Check sheet for the modelled part. Datum: model origin and axes. Units: mm. A direction names the side the tool comes from. Round coordinates to 2 decimals unless told otherwise and drop trailing zeros. Loops run counter-clockwise (first coordinate to the right, second up) from the corner with the lowest first, then second, coordinate; pieces in that order, holes last. Notation, with made-up numbers: (-2, 32.25) -> (24, 32.25) arc R5 cw to (24, 41.25) -> close; hole circle Ø7 at (64, 89.25). An arc over 180 degrees is marked (long way). Return JSON: item names as keys, results as strings.
from build123d import *

# Parameters (mm, degrees)
ESQUISSE1_W             = 49.5
ESQUISSE1_H             = 49.5
ESQUISSE1_W_2           = 43.5
ESQUISSE1_H_2           = 43.5
BOSS_EXTRU_1_DEPTH      = 30
ESQUISSE2_W             = 10
ESQUISSE2_H             = 10
ESQUISSE2_R             = 1.75
BOSS_EXTRU_2_DEPTH      = 5
CONG_1_R                = 1
CONG_2_R                = 3
CONG_3_R                = 1
CUT_EXTRUDE1_DEPTH      = 24
CUT_EXTRUDE1_DEPTH_BACK = 21.171554026
SKETCH1_W               = 3.5
SKETCH1_H               = 15


with BuildPart() as part:
    # Esquisse1 → Boss.-Extru.1 (new body)
    with BuildSketch(Plane.XY):
        with Locations((24.75, 24.75)):
            Rectangle(ESQUISSE1_W, ESQUISSE1_H)
        with Locations((24.75, 24.75)):
            Rectangle(ESQUISSE1_W_2, ESQUISSE1_H_2, mode=Mode.SUBTRACT)
    extrude(amount=BOSS_EXTRU_1_DEPTH)

    # Esquisse2 → Boss.-Extru.2 (add)
    # profile 1 of 2: a face of its own
    with BuildSketch(Plane(origin=(0, 0, 0), x_dir=(-1, 0, 0), z_dir=(0, 0, -1))):
        with Locations((-5, 54.5)):
            Rectangle(ESQUISSE2_W, ESQUISSE2_H)
        with Locations((-5, 54.5)):
            Circle(ESQUISSE2_R, mode=Mode.SUBTRACT)
    # profile 2 of 2: a face of its own
    with BuildSketch(Plane(origin=(0, 0, 0), x_dir=(-1, 0, 0), z_dir=(0, 0, -1))):
        with Locations((-44.5, -5)):
            Rectangle(ESQUISSE2_W, ESQUISSE2_H)
        with Locations((-44.5, -5)):
            Circle(ESQUISSE2_R, mode=Mode.SUBTRACT)
    extrude(amount=-BOSS_EXTRU_2_DEPTH)

    # Congé1
    cong_1_edges = [part.edges().sort_by_distance(p)[0] for p in [
        (0, 59.5, 2.5),
        (10, 59.5, 2.5),
        (49.5, -10, 2.5),
        (39.5, -10, 2.5),
        (49.5, 49.5, 15),
        (0, 0, 15),
    ]]
    fillet(cong_1_edges, radius=CONG_1_R)

    # Congé2
    cong_2_edges = [part.edges().sort_by_distance(p)[0] for p in [
        (10, 49.5, 2.5),
        (39.5, 0, 2.5),
    ]]
    fillet(cong_2_edges, radius=CONG_2_R)

    # Congé3
    cong_3_edges = [part.edges().sort_by_distance(p)[0] for p in [
        (6.5, 49.5, 5),
        (43, 0, 5),
    ]]
    fillet(cong_3_edges, radius=CONG_3_R)

    # Sketch1 → Cut-Extrude1 (cut, two sides: drawn at the far end of the back side and taken through both)
    with BuildSketch(Plane.XZ.offset(-CUT_EXTRUDE1_DEPTH_BACK)):
        with BuildLine():
            ThreePointArc((28.75, 15), (25.25, 18.5), (21.75, 15))
            Line((21.75, 15), (25.25, 15))
            Line((25.25, 15), (28.75, 15))
        make_face()
        with Locations((27, 7.5)):
            Rectangle(SKETCH1_W, SKETCH1_H)
        with Locations((23.5, 7.5)):
            Rectangle(SKETCH1_W, SKETCH1_H)
    extrude(amount=CUT_EXTRUDE1_DEPTH + CUT_EXTRUDE1_DEPTH_BACK, mode=Mode.SUBTRACT)


solid = part.part
Q1. Section check C-C (x = 44.5). Record the boundary of the cut face in (y, z).
Results list:
{"outline": "(-10, 0) -> (-6.75, 0) -> (-6.75, 5) -> (-10, 5) -> close; (-3.25, 0) -> (3, 0) -> (3, 30) -> (0, 30) -> (0, 6) arc R1 cw to (-1, 5) -> (-3.25, 5) -> close; (46.5, 0) -> (49.5, 0) -> (49.5, 30) -> (46.5, 30) -> close"}
Q2. Go/stop test with flat-tipped pins: pin 1 (15 mm diameter, centred on x = 13.5, z = 17, fed in from -Y); pin 2 (1 mm diameter, centred on x = 29.5, z = 14.5, fed in from +Y); pin 3 (2 mm diameter, centred on x = 5, y = 54.5, fed in from -Z); pin 4 (7 mm diameter, centred on x = 5.5, y = 54.5, fed in from +Z). Record where each tip stops, or that it passes through.
Results list:
{"pin 1": "y = 0", "pin 2": "y = 49.5", "pin 3": "through", "pin 4": "z = 5"}
Q3. Draft check along X on faces 5 (the flat face through (39.5, -6, 2)), 6 (the flat face through (25, 48, 0)), 7 (the flat face through (3, 24, 15)), 8 (the flat face through (49.5, 19, 15)). Enter one of: released by +X, released by -X, zero draft, split by the parting line, or undercut.
Results list:
{"face 5": "released by -X", "face 6": "zero draft", "face 7": "undercut", "face 8": "released by +X"}
Q4. Section check A-A (x = 21). Record the boundary of the cut face in (y, z), then the cut area to 3 significant figures.
Results list:
{"outline": "(0, 0) -> (3, 0) -> (3, 30) -> (0, 30) -> close; (46.5, 0) -> (49.5, 0) -> (49.5, 30) -> (46.5, 30) -> close", "area": "180 mm^2"}
Q5. Section check D-D (z = 12.5). Record the boundary of the cut face in (x, y).
Results list:
{"outline": "(0, 1) arc R1 ccw to (1, 0) -> (21.75, 0) -> (21.75, 3) -> (3, 3) -> (3, 46.5) -> (46.5, 46.5) -> (46.5, 3) -> (28.75, 3) -> (28.75, 0) -> (49.5, 0) -> (49.5, 48.5) arc R1 ccw to (48.5, 49.5) -> (0, 49.5) -> close"}
Q6. Material ranges on line 1 (Y direction, x = 44.5, z = 2.5); line 2 (Y direction, x = 5, z = 1); line 3 (Y direction, x = 32, z = 15), recorded low to high.
Results list:
{"line 1": "-10 to -6.75, -3.25 to 3, 46.5 to 49.5", "line 2": "0 to 3, 46.5 to 52.75, 56.25 to 59.5", "line 3": "0 to 3, 46.5 to 49.5"}
Q7. Tool access check on faces 1 (the flat face through (47, -5, 5)), 2 (the flat face through (28.75, 2, 7)), 3 (the flat face through (3, 55, 5)), 4 (the flat face through (10, 55, 2)). Record the directions out of +Z, -Z, +X, -X, +Y, -Y that give a thin tool (end or side, any length) a straight path to the whole face; none if there is none.
Results list:
{"face 1": "+Z, +X, -X, -Y", "face 2": "-Z, -Y", "face 3": "+Z, +X, -X, +Y", "face 4": "+Z, -Z, +X, +Y"}
Q8. Section check B-B (y = 54.5). Record the boundary of the cut face in (x, z), then the cut area to 3 significant figures.
Results list:
{"outline": "(0, 0) -> (3.25, 0) -> (3.25, 5) -> (0, 5) -> close; (6.75, 0) -> (10, 0) -> (10, 5) -> (6.75, 5) -> close", "area": "32.5 mm^2"}
